```python
from build123d import *

# Parameters (mm, degrees)
SKETCH1_R           = 2
SKETCH1_R_2         = 4
SKETCH1_R_3         = 1.5
SKETCH1_W           = 5
SKETCH1_H           = 10
BOSS_EXTRUDE1_DEPTH = 5


with BuildPart() as part:
    # Sketch1 → Boss-Extrude1 (new body)
    with BuildSketch(Plane.XY):
        with BuildLine():
            Line((-30, 19.5), (30, 19.5))
            ThreePointArc((30, 19.5), (49.5, 0), (30, -19.5))
            Line((30, -19.5), (-30, -19.5))
            ThreePointArc((-30, -19.5), (-49.5, 0), (-30, 19.5))
        make_face()
        with Locations((-30, 12)):
            Circle(SKETCH1_R, mode=Mode.SUBTRACT)
        with Locations((-18, 0)):
            Circle(SKETCH1_R, mode=Mode.SUBTRACT)
        with Locations((-30, -12)):
            Circle(SKETCH1_R, mode=Mode.SUBTRACT)
        with Locations((-42, 0)):
            Circle(SKETCH1_R, mode=Mode.SUBTRACT)
        with Locations((-30, 0)):
            Circle(SKETCH1_R_2, mode=Mode.SUBTRACT)
        with Locations((15, 12)):
            Circle(SKETCH1_R_3, mode=Mode.SUBTRACT)
        with Locations((15, -12)):
            Circle(SKETCH1_R_3, mode=Mode.SUBTRACT)
        with BuildLine():
            Line((15, -5), (0, -5))
            ThreePointArc((0, -5), (-5, 0), (0, 5))
            Line((0, 5), (15, 5))
            ThreePointArc((15, 5), (20, 0), (15, -5))
        make_face(mode=Mode.SUBTRACT)
        with Locations((30, 9.5)):
            Rectangle(SKETCH1_W, SKETCH1_H, mode=Mode.SUBTRACT)
        with Locations((30, -9.5)):
            Rectangle(SKETCH1_W, SKETCH1_H, mode=Mode.SUBTRACT)
        with BuildLine():
            ThreePointArc((-11.950316083, 6.944527868), (-11.782969997, 8.348805364), (-10.3786925, 8.181459278))
            ThreePointArc((-10.3786925, 8.181459278), (-8.018515434, 2.995451326), (-8.316401238, -2.694573131))
            ThreePointArc((-8.316401238, -2.694573131), (-9.561940964, -3.364372198), (-10.231740032, -2.118832472))
            ThreePointArc((-10.231740032, -2.118832472), (-9.983501861, 2.622854574), (-11.950316083, 6.944527868))
        make_face(mode=Mode.SUBTRACT)
    extrude(amount=BOSS_EXTRUDE1_DEPTH)


solid = part.part
```
Input: part model. Units: mm. Frame: model coordinates. A direction names the side the tool comes from. Give positions to 0.01 mm unless a question says otherwise; leave off trailing zeros. Write each loop counter-clockwise with the first axis right and the second up, starting at its lowest first coordinate (ties: lowest second). Pieces come first, ordered by that corner, then holes. Notation, with made-up numbers: (-39, 1) - (-6, 1) arc R8 cw to (-6, 10) - close; hole circle Ø3 at (-23, 62.5). An arc over 180 degrees is marked (long way). Write item = value, one per line. Start each with the question number.
1. Section query B-B, the plane y = 3. Output: boundary loops of the cut face in (x, z).
2. First-contact query: pin 1 Ø3 at (x, y) = (-42, 0) entering from +Z; pin 2 Ø12 at (x, y) = (8, 4.5) entering from -Z; pin 3 Ø1.5 at (x, z) = (37.5, 0.5) entering from -Y; pin 4 Ø1.5 at (y, z) = (-8.5, 3) entering from +X. Flat tips, straight axial feed; report the tip coordinate or a pass-through.
3. Section query A-A, the plane x = 2. Output: boundary loops of the cut face in (y, z), then the cut area to 3 significant figures.
4. Mould query, pull axis Y, two halves, no side actions, for faces 3 (the flat face through (1, -8, 0)), 4 (the flat face through (27.5, -10, 2)), 5 (the flat face through (0, 19.5, 2)). Classes: released by +Y, released by -Y, zero draft, split by the parting line, or undercut.
5. Section query D-D, the plane y = -12. Output: boundary loops of the cut face in (x, z), then the cut area to 3 significant figures.
6. Ray query, L1, parallel to Y at x = 28.5, z = 1.85; L2, parallel to Y at x = -30, z = 2.7; L3, parallel to Y at x = 5.5, z = 2.7. Return the intervals inside material, ascending.
7. Access query for faces 1 (the flat face through (1, -8, 5)), 2 (the cylindrical face through (-9.97, 2.56, 2.46)). Directions: +Z, -Z, +X, -X, +Y, -Y. A direction counts if a zero-diameter tool reaches every point of the face in a straight line with its end or side. Return the directions, or none.
8. Section query C-C, the plane z = 4.25. Count the separate pieces of the cut face and the enclosed holes in it, then the cut area to 3 significant figures.
Check sheet entries:
q1.outline = (-49.27, 0) - (-32.65, 0) - (-32.65, 5) - (-49.27, 5) - close; (-27.35, 0) - (-10.06, 0) - (-10.06, 5) - (-27.35, 5) - close; (-8.02, 0) - (-4, 0) - (-4, 5) - (-8.02, 5) - close; (19, 0) - (49.27, 0) - (49.27, 5) - (19, 5) - close
q2.pin_1 = through
q2.pin_2 = 0
q2.pin_3 = -18.29
q2.pin_4 = 47.89
q3.outline = (-19.5, 0) - (-5, 0) - (-5, 5) - (-19.5, 5) - close; (5, 0) - (19.5, 0) - (19.5, 5) - (5, 5) - close
q3.area = 145 mm2
q4.face_3 = zero draft
q4.face_4 = undercut
q4.face_5 = released by +Y
q5.outline = (-45.37, 0) - (-32, 0) - (-32, 5) - (-45.37, 5) - close; (-28, 0) - (13.5, 0) - (13.5, 5) - (-28, 5) - close; (16.5, 0) - (27.5, 0) - (27.5, 5) - (16.5, 5) - close; (32.5, 0) - (45.37, 0) - (45.37, 5) - (32.5, 5) - close
q5.area = 394 mm2
q6.L1 = -19.5 to -14.5, -4.5 to 4.5, 14.5 to 19.5
q6.L2 = -19.5 to -14, -10 to -4, 4 to 10, 14 to 19.5
q6.L3 = -19.5 to -5, 5 to 19.5
q7.face_1 = +Z, +X, -X, +Y, -Y
q7.face_2 = +Z, -Z
q8.separate_pieces = 1
q8.enclosed_holes = 11
q8.area = 3,070 mm2
